Design review of the part built by this model. Coordinates are the model's own, in mm. Coordinates: 2 decimals unless noted, no trailing zeros. Order: outer loops, then holes, each group sorted by start corner. A loop starts at its lowest first (then second) coordinate and runs counter-clockwise, first axis right, second up.
from build123d import *

# Parameters (mm, degrees)
F0_W     = 25.4
F0_H     = 2.54
F1_DEPTH = 2.54


with BuildPart() as f1:
    # F0 (on Front) → F1 (new body)
    with BuildSketch(Plane.XZ):
        Polygon((0, 86.929028), (-10.90126, 63.987308), (-21.80252, 41.045588), (-32.703781, 18.103867), (-43.605041, -4.837853), (-54.562222, -27.897259), (-65.463482, -50.838979), (-76.364742, -73.780699), (-50.964742, -73.780699), (-25.564742, -73.780699), (-0.152042, -73.780699), (25.247958, -73.780699), (50.647958, -73.780699), (76.060658, -73.780699), (65.19485, -50.822167), (54.329041, -27.863634), (43.463233, -4.905102), (32.597425, 18.053431), (21.731617, 41.011963), (10.865808, 63.970496), align=None)
        Polygon((-13.195432, 65.077434), (-10.90126, 63.987308), (0, 86.929028), (-2.294172, 88.019154), align=None)
        Polygon((-32.703781, 18.103867), (-21.80252, 41.045588), (-24.096692, 42.135714), (-34.997953, 19.193993), align=None)
        Polygon((13.161662, 65.057076), (10.865808, 63.970496), (21.731617, 41.011963), (24.02747, 42.098544), align=None)
        Polygon((-54.562222, -27.897259), (-43.605041, -4.837853), (-45.272266, -4.189892), (-56.173526, -27.131612), align=None)
        Polygon((34.893278, 19.140012), (32.597425, 18.053431), (43.463233, -4.905102), (45.759086, -3.818521), align=None)
        Polygon((-76.364742, -73.780699), (-65.463482, -50.838979), (-67.757654, -49.748853), (-78.658914, -72.690573), align=None)
        Polygon((56.624895, -26.777053), (54.329041, -27.863634), (65.19485, -50.822167), (67.490703, -49.735586), align=None)
        with Locations((-38.264742, -75.050699)):
            Rectangle(F0_W, F0_H)
        Polygon((76.047958, -76.320699), (76.060658, -73.780699), (50.647958, -73.780699), (50.647958, -76.320699), align=None)
        with Locations((12.547958, -75.050699)):
            Rectangle(F0_W, F0_H)
    extrude(amount=F1_DEPTH)


solid = f1.part
1. Add section B-B (x = -19). Give the boundary of the cut face in (y, z).
2. To check wall thickness, follow line 1 (X direction, y = -1, z = 42); line 2 (Z direction, x = 23, y = -2.1); line 3 (X direction, y = -0.2, z = 18.5). State the ranges of each line that lie inside material, in increasing order.
3. Add section A-A (z = 54). Give the boundary of the cut face in (x, y), and give its area (3 significant figures).
4. Mouldability with a two-part tool opening along Z and no side actions: class faces 1 (the flat face through (40.402, -1.252, 7.5)), 2 (the flat face through (-2, -2.54, -11)), 3 (the flat face through (70.704, -1.252, -62.462)) as pulls with the +Z half, pulls with the -Z half, needs draft (parallel to the pull), parting line crosses it, or undercut.
5. Insertion check: pin 1 (4 mm diameter, centred on x = 2, z = -16, fed in from +Y); pin 2 (1.3 mm diameter, centred on y = -1, z = -75.5, fed in from -X); pin 3 (0.8 mm diameter, centred on x = -6.5, y = -1.5, fed in from -Z). Each pin has a flat end and moves straight along its axis. Give the tip position at first contact, or say it passes through.
Solution:
1. outline: (-2.54, -73.78) - (0, -73.78) - (0, 46.94) - (-2.54, 46.94) - close
2. line 1: x = -24.16 to -23.81, -21.35 to 23.82
2. line 2: z = -76.32 to 38.33, 41.61 to 44.27
2. line 3: x = -33.54 to 32.39, 33.54 to 35.2
3. outline: (-15.65, -2.54) - (18.39, -2.54) - (18.39, 0) - (-15.65, 0) - close
3. area: 86.5 mm2
4. face 1: pulls with the +Z half
4. face 2: needs draft
4. face 3: undercut
5. pin 1: stops at y = 0
5. pin 2: stops at x = -50.96
5. pin 3: stops at z = -73.78
